```python
from build123d import *

# Parameters (mm, degrees)
SKETCH_1_W            = 15
SKETCH_1_H            = 20
EXTRUDE_1_DEPTH       = 15
SKETCH_2_W            = 12
SKETCH_2_H            = 12
CUT_EXTRUDE_1_DEPTH   = 30.154759474
HOLE_WIZARD_3_0_3_1_D = 3
HOLE_WIZARD_3_0_3_2_D = 3
FILLET_1_R            = 5


with BuildPart() as part:
    # 草图1 → 凸台-拉伸1 (new body)
    with BuildSketch(Plane(origin=(0, 0, 0), x_dir=(1, 0, 0), z_dir=(0, 1, 0))):
        with Locations((7.5, -10)):
            Rectangle(SKETCH_1_W, SKETCH_1_H)
    extrude(amount=-EXTRUDE_1_DEPTH)

    # 草图2 → 切除-拉伸1 (cut, through all)
    with BuildSketch(Plane(origin=(0, 0, 0), x_dir=(-1, 0, 0), z_dir=(0, 0, -1))):
        with Locations((-9, -6)):
            Rectangle(SKETCH_2_W, SKETCH_2_H)
    extrude(amount=-CUT_EXTRUDE_1_DEPTH, mode=Mode.SUBTRACT)

    # Ø3.0 (3) 直径孔1 (through all)
    with Locations(Plane(origin=(3, 0, 0), x_dir=(0, 0, -1), z_dir=(1, 0, 0))):
        with Locations((-5, -5), (-15, -5)):
            Hole(HOLE_WIZARD_3_0_3_1_D / 2)

    # Ø3.0 (3) 直径孔2 (through all)
    with Locations(Plane(origin=(0, -12, 0), x_dir=(1, 0, 0), z_dir=(0, 1, 0))):
        with Locations((10, -5), (10, -15)):
            Hole(HOLE_WIZARD_3_0_3_2_D / 2)

    # 圆角1
    fillet_1_edges = [part.edges().sort_by_distance(p)[0] for p in [
        (3, -12, 10),
    ]]
    fillet(fillet_1_edges, radius=FILLET_1_R)


solid = part.part
```
Can you work these out from the model? Positions are in its coordinate system, mm. A direction names the side the tool comes from. Give positions to 0.01 mm unless a question says otherwise; leave off trailing zeros. Write each loop counter-clockwise with the first axis right and the second up, starting at its lowest first coordinate (ties: lowest second). Pieces come first, ordered by that corner, then holes. Notation, with made-up numbers: (54, -11.5) - (98, -11.5) arc R9 ccw to (98, -3.5) - close; hole circle Ø11 at (-0.5, 38.5). An arc over 180 degrees is marked (long way). Write item = value, one per line. Start each with the question number.
1. Imagine slicing it at B-B (y = -5). Please give me the cut outline in (x, z), and give its area (3 significant figures).
2. Imagine slicing it at D-D (z = 8.75). Please give me the cut outline in (x, y).
3. Imagine slicing it at A-A (z = 5). Please give me the cut outline in (x, y).
4. For pin 1 (3 mm diameter, centred on x = 11.5, z = 2.5, fed in from +Y); pin 2 (6 mm diameter, centred on y = -8.5, z = 4.5, fed in from +X); pin 3 (1.8 mm diameter, centred on x = 10, z = 5, fed in from +Y); pin 4 (1 mm diameter, centred on y = -3.5, z = 4.5, fed in from +X), each with a flat end and sliding along its axis, tell me the tip position at first contact or that it passes through.
5. Thinking about a two-plate mould opening in X: for faces 3 (the face through (4, -10, 10)), 4 (the face through (11.5, -13.52, 4.93)), 5 (the face through (1, 0, 10)), which applies, released by +X, released by -X, zero draft, split by the parting line, or undercut?
6. Please list where these lines run through material, in increasing order: line 1 (Z direction, x = 10, y = -13.4); line 2 (Y direction, x = 1.1, z = 15); line 3 (Y direction, x = 13, z = 10.5).
7. Imagine slicing it at C-C (x = 10). Please give me the cut outline in (y, z), and give its area (3 significant figures).
8. On a 3-axis mill with a long thin cutter (end or side, diameter ignored), from which of +Z, -Z, +X, -X, +Y, -Y can I reach the whole of each face in a straight line? I mean faces 1 (the face through (1.479, -3.735, 5.806)), 2 (the face through (12, -12, 10)). Say none if no direction works.
Worked answers:
q1.outline = (0, 0) - (3, 0) - (3, 3.5) - (0, 3.5) - close; (0, 6.5) - (3, 6.5) - (3, 13.5) - (0, 13.5) - close; (0, 16.5) - (3, 16.5) - (3, 20) - (0, 20) - close
q1.area = 42.0 mm2
q2.outline = (0, -15) - (15, -15) - (15, -12) - (8, -12) arc R5 cw to (3, -7) - (3, 0) - (0, 0) - close
q3.outline = (0, -15) - (8.5, -15) - (8.5, -12) - (8, -12) arc R5 cw to (3, -7) - (3, -6.5) - (0, -6.5) - close; (0, -3.5) - (3, -3.5) - (3, 0) - (0, 0) - close; (11.5, -15) - (15, -15) - (15, -12) - (11.5, -12) - close
q4.pin_1 = -12
q4.pin_2 = 5.82
q4.pin_3 = through
q4.pin_4 = 3
q5.face_3 = released by +X
q5.face_4 = undercut
q5.face_5 = zero draft
q6.line_1 = 0 to 3.5, 6.5 to 13.5, 16.5 to 20
q6.line_2 = -15 to -6.5, -3.5 to 0
q6.line_3 = -15 to -12
q7.outline = (-15, 0) - (-12, 0) - (-12, 3.5) - (-15, 3.5) - close; (-15, 6.5) - (-12, 6.5) - (-12, 13.5) - (-15, 13.5) - close; (-15, 16.5) - (-12, 16.5) - (-12, 20) - (-15, 20) - close
q7.area = 42.0 mm2
q8.face_1 = +X, -X
q8.face_2 = +Z, -Z, +X, +Y
